Check sheet for the modelled part. Datum: model origin and axes. Units: mm. Face numbers are marked on the shaded views. A direction names the side the tool comes from. Give positions to 0.01 mm unless a question says otherwise; leave off trailing zeros. Loops run counter-clockwise (first coordinate to the right, second up) from the corner with the lowest first, then second, coordinate; pieces in that order, holes last. Notation, with made-up numbers: (2.5, -15.5) -> (6.5, -15.5) arc R26 ccw to (6.5, -1.5) -> close; hole circle Ø2 at (63.25, 70.25). An arc over 180 degrees is marked (long way). Write each question's results on one line, items separated by ' | '. Start each with the question number.
1. Cross-section at C-C on x = 1.5. Record the boundary of the cut face in (y, z).
2. Material ranges on L1, parallel to X at y = 2.5, z = -0.25; L2, parallel to Y at x = 6, z = -1.5, recorded low to high. Write a range as from..to.
3. Cross-section at B-B on z = -5.75. Record the boundary of the cut face in (x, y), and give its area (3 significant figures).
4. Cross-section at A-A on y = 4.5. Record the boundary of the cut face in (x, z), and give its area (3 significant figures).
5. Mould release check, pull along Z, two halves, no side actions. Record for the marked faces 1, 2, 3 and 4: +Z half, -Z half, draft (parallel to the pull), parting line (faces both ways), or undercut.
6. Tool access check on the marked faces 5 and 6. Record the directions out of +Z, -Z, +X, -X, +Y, -Y that give a thin tool (end or side, any length) a straight path to the whole face; none if there is none.
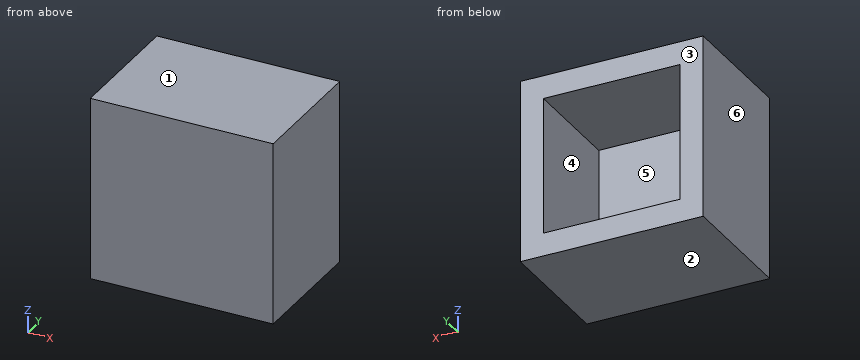
Autodesk Inventor part; units mm, degrees
ref_plane "YZ Plane" through (0, 0, 0) normal (1, 0, 0) x (0, 1, 0)
ref_plane "XZ Plane" through (0, 0, 0) normal (0, 1, 0) x (-1, 0, 0)
ref_plane "XY Plane" through (0, 0, 0) normal (0, 0, 1) x (1, 0, 0)
sketch "Sketch1" plane through (0, 0, 0) normal (0, 1, 0) x (-1, 0, 0)
  line L0 (-8.5, 8.5) -> (8.5, 8.5)
  line L1 (8.5, 8.5) -> (8.5, -8.5)
  line L2 (8.5, -8.5) -> (-8.5, -8.5)
  line L3 (-8.5, -8.5) -> (-8.5, 8.5)
  line L4 (-8.5, 8.5) -> (8.5, -8.5) construction
  line L5 (8.5, 8.5) -> (-8.5, -8.5) construction
  point P0 (0, 0)
  dimension "d0" = 17
  dimension "d1" = 17
extrude "Extrusion1" add sketch "Sketch1" along normal blind 2
sketch "Sketch2" plane through (0, 2, 0) normal (0, 1, 0) x (1, 0, 0)
  line L0 (8.5, 8.5) -> (-8.5, 8.5)
  line L1 (8.5, -8.5) -> (-8.5, -8.5)
  line L2 (-8.5, -8.5) -> (-8.5, 8.5)
  line L3 (-8.5, 8.5) -> (8.5, 8.5)
  line L4 (8.5, 8.5) -> (8.5, -8.5)
  line L5 (8.5, -8.5) -> (-8.5, 8.5) construction
  line L6 (-8.5, -8.5) -> (8.5, 8.5) construction
  line L7 (6.35, -6.35) -> (-6.35, -6.35)
  line L8 (-6.35, -6.35) -> (-6.35, 6.35)
  line L9 (-6.35, 6.35) -> (6.35, 6.35)
  line L10 (6.35, 6.35) -> (6.35, -6.35)
  line L11 (6.35, -6.35) -> (-6.35, 6.35) construction
  line L12 (-6.35, -6.35) -> (6.35, 6.35) construction
  point P0 (0, 0)
  dimension "d4" = 12.7
extrude "Extrusion2" add sketch "Sketch2" along normal blind 10
properties part number "bar_protector" material "Rubber, Butyl"
Geometry says:
1) outline: (0, -8.5) -> (12, -8.5) -> (12, -6.35) -> (2, -6.35) -> (2, 6.35) -> (12, 6.35) -> (12, 8.5) -> (0, 8.5) -> close
2) L1: -8.5..-6.35, 6.35..8.5 | L2: 0..2
3) outline: (-8.5, 0) -> (8.5, 0) -> (8.5, 12) -> (6.35, 12) -> (6.35, 2) -> (-6.35, 2) -> (-6.35, 12) -> (-8.5, 12) -> close | area: 77.0 mm^2
4) outline: (-8.5, -8.5) -> (8.5, -8.5) -> (8.5, 8.5) -> (-8.5, 8.5) -> close; hole (-6.35, -6.35) -> (6.35, -6.35) -> (6.35, 6.35) -> (-6.35, 6.35) -> close | area: 128 mm^2
5) face 1: +Z half | face 2: -Z half | face 3: draft | face 4: undercut
6) face 5: +Y | face 6: +Z, -Z, -X, +Y, -Y
